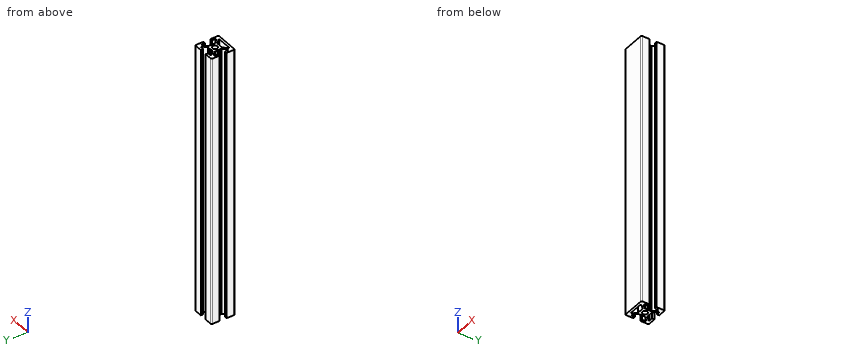
Autodesk Inventor part; units mm, degrees
ref_plane "C1_XY" through (0, 0, 0) normal (0, 0, 1) x (1, 0, 0)
ref_plane "C1_YZ" through (0, 0, 0) normal (1, 0, 0) x (0, 1, 0)
ref_plane "C1_ZX" through (0, 0, 0) normal (0, 1, 0) x (0, 0, 1)
sketch "Sketch_76" plane through (0, 0, 0) normal (0, 0, 1) x (1, 0, 0)
  line L0 (-10, -3) -> (-10, -9)
  arc A0 (-10, -9) -> (-9, -10) centre (-9, -9) ccw
  line L1 (-9, -10) -> (9, -10)
  arc A1 (9, -10) -> (10, -9) centre (9, -9) ccw
  line L2 (10, -9) -> (10, -3)
  line L3 (10, -3) -> (8, -3)
  line L4 (8, -3) -> (8, -6)
  line L5 (8, -6) -> (7.0607, -6)
  line L6 (7.0607, -6) -> (4, -2.9393)
  line L7 (4, -2.9393) -> (4, -0.6536)
  arc A2 (4, -0.6536) -> (3.933, -0.4036) centre (3.5, -0.6536) ccw
  line L8 (3.933, -0.4036) -> (3.7, 0)
  line L9 (3.7, 0) -> (3.933, 0.4036)
  arc A3 (3.933, 0.4036) -> (3.933, 0.9036) centre (3.5, 0.6536) ccw
  line L10 (3.933, 0.9036) -> (3.751, 1.2189)
  line L11 (3.751, 1.2189) -> (4, 2.5)
  line L12 (4, 2.5) -> (4, 2.9393)
  line L13 (4, 2.9393) -> (7.0607, 6)
  line L14 (7.0607, 6) -> (8, 6)
  line L15 (8, 6) -> (8, 3)
  line L16 (8, 3) -> (10, 3)
  line L17 (10, 3) -> (10, 9)
  arc A4 (10, 9) -> (9, 10) centre (9, 9) ccw
  line L18 (9, 10) -> (3, 10)
  line L19 (3, 10) -> (3, 8)
  line L20 (3, 8) -> (6, 8)
  line L21 (6, 8) -> (6, 7.0607)
  line L22 (6, 7.0607) -> (2.9393, 4)
  line L23 (2.9393, 4) -> (0.6536, 4)
  arc A5 (0.6536, 4) -> (0.4036, 3.933) centre (0.6536, 3.5) ccw
  line L24 (0.4036, 3.933) -> (0, 3.7)
  line L25 (0, 3.7) -> (-0.4036, 3.933)
  arc A6 (-0.4036, 3.933) -> (-0.9036, 3.933) centre (-0.6536, 3.5) ccw
  line L26 (-0.9036, 3.933) -> (-1.2189, 3.751)
  line L27 (-1.2189, 3.751) -> (-2.5, 4)
  line L28 (-2.5, 4) -> (-2.9393, 4)
  line L29 (-2.9393, 4) -> (-6, 7.0607)
  line L30 (-6, 7.0607) -> (-6, 8)
  line L31 (-6, 8) -> (-3, 8)
  line L32 (-3, 8) -> (-3, 10)
  line L33 (-3, 10) -> (-9, 10)
  arc A7 (-9, 10) -> (-10, 9) centre (-9, 9) ccw
  line L34 (-10, 9) -> (-10, 3)
  line L35 (-10, 3) -> (-8, 3)
  line L36 (-8, 3) -> (-8, 6)
  line L37 (-8, 6) -> (-7.0607, 6)
  line L38 (-7.0607, 6) -> (-4, 2.9393)
  line L39 (-4, 2.9393) -> (-4, 0.6536)
  arc A8 (-4, 0.6536) -> (-3.933, 0.4036) centre (-3.5, 0.6536) ccw
  line L40 (-3.933, 0.4036) -> (-3.7, 0)
  line L41 (-3.7, 0) -> (-3.933, -0.4036)
  arc A9 (-3.933, -0.4036) -> (-3.933, -0.9036) centre (-3.5, -0.6536) ccw
  line L42 (-3.933, -0.9036) -> (-3.751, -1.2189)
  line L43 (-3.751, -1.2189) -> (-4, -2.5)
  line L44 (-4, -2.5) -> (-4, -2.9393)
  line L45 (-4, -2.9393) -> (-7.0607, -6)
  line L46 (-7.0607, -6) -> (-8, -6)
  line L47 (-8, -6) -> (-8, -3)
  line L48 (-8, -3) -> (-10, -3)
  line L49 (-6, -7.2678) -> (-6, -7.5)
  arc A10 (-6, -7.5) -> (-5.5, -8) centre (-5.5, -7.5) ccw
  line L50 (-5.5, -8) -> (5.5, -8)
  arc A11 (5.5, -8) -> (6, -7.5) centre (5.5, -7.5) ccw
  line L51 (6, -7.5) -> (6, -7.2678)
  arc A12 (6, -7.2678) -> (5.8536, -6.9142) centre (5.5, -7.2678) ccw
  line L52 (5.8536, -6.9142) -> (3.0858, -4.1464)
  arc A13 (3.0858, -4.1464) -> (2.7322, -4) centre (2.7322, -4.5) ccw
  line L53 (2.7322, -4) -> (-2.7322, -4)
  arc A14 (-2.7322, -4) -> (-3.0858, -4.1464) centre (-2.7322, -4.5) ccw
  line L54 (-3.0858, -4.1464) -> (-5.8536, -6.9142)
  arc A15 (-5.8536, -6.9142) -> (-6, -7.2678) centre (-5.5, -7.2678) ccw
extrude "Extrusion1" add sketch "Sketch_76" against normal blind 230
sketch "Sketch2" plane through (0, 0, -230) normal (0, 0, -1) x (-1, 0, 0)
  point P0 (0, 0)
hole "Hole1" at (0, 0, -230) direction (0, 0, 1) diameter 4.2 depth 230
ref_plane "C1_XY" through (0, 0, 0) normal (0, 0, 1) x (1, 0, 0)
ref_plane "C1_YZ" through (0, 0, 0) normal (1, 0, 0) x (0, 1, 0)
ref_plane "C1_ZX" through (0, 0, 0) normal (0, 1, 0) x (0, 0, 1)
properties part number "NFSF5-2020-230"
Geometry: final body of the model. Coordinates: model frame, mm. Round coordinates to 2 decimals unless told otherwise and drop trailing zeros.
Item 1: Material intervals for L1, parallel to Y at x = 0, z = -175.5; L2, parallel to Y at x = 4.5, z = -12.5; L3, parallel to Y at x = -1.5, z = -113, sorted ascending.
Item 2: Pin query (flat end, axial travel): P1, Ø4, axis at y = 2, z = -53, coming from the +X side; P2, Ø2, axis at y = 0.5, z = -107, coming from the +X side; P3, Ø1.5, axis at x = -0.5, z = -96.5, coming from the +Y side. Return the tip coordinate at first contact, or that it passes through.
Item 3: Section query A-A (z = -75). Give the number of separate pieces and of enclosed holes in the cut face, plus the area to 3 significant figures.
Completed:
1. L1: y = -10 to -8, -4 to -2.1, 2.1 to 3.7
1. L2: y = -10 to -8, -5.56 to -3.44, 3.44 to 5.56, 8 to 10
1. L3: y = -10 to -8, -4 to -1.47, 1.47 to 3.81
2. P1: stops at x = 10
2. P2: stops at x = 4
2. P3: stops at y = 4
3. separate pieces: 1
3. enclosed holes: 2
3. area: 194 mm2
